CAD build for the part. Positions are in the model's coordinates, mm. Round coordinates to 2 decimals unless told otherwise and drop trailing zeros. Write each loop counter-clockwise with the first axis right and the second up, starting at its lowest first coordinate (ties: lowest second). Pieces come first, ordered by that corner, then holes. Notation, with made-up numbers: (46, 42) - (92, 42) arc R24 cw to (92, 57) - close; hole circle Ø11 at (52.25, -15). An arc over 180 degrees is marked (long way). Answer in a Markdown table with one row per item.
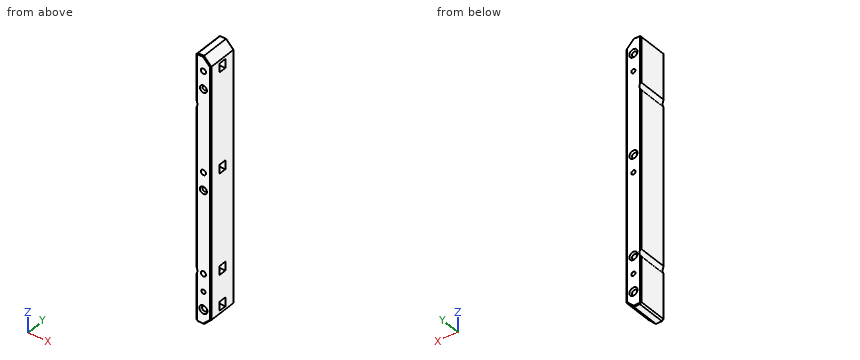
```python
from build123d import *

# Parameters (mm, degrees)
SKETCH1_W           = 10
SKETCH1_H           = 20
BOSS_EXTRUDE1_DEPTH = 90
SKETCH6_R           = 1.75
CUT_EXTRUDE4_DEPTH  = 93.330926563
SKETCH7_R           = 1.4
CUT_EXTRUDE5_DEPTH  = 93.330926563
CUT_EXTRUDE6_START  = -10
CUT_EXTRUDE6_DEPTH  = 2.5
CHAMFER2_SIZE       = 5
CHAMFER3_SIZE       = 1
CHAMFER4_SIZE       = 0.5
CHAMFER5_SIZE       = 0.5
SKETCH10_R          = 3.75
CUT_EXTRUDE7_DEPTH  = 93.330926563


with BuildPart() as part:
    # Sketch1 → Boss-Extrude1 (new, symmetric)
    with BuildSketch(Plane.XY):
        Rectangle(SKETCH1_W, SKETCH1_H)
    extrude(amount=BOSS_EXTRUDE1_DEPTH, both=True)

    # Sketch6 → Cut-Extrude4 (cut, through all)
    with BuildSketch(Plane.XZ.offset(10)):
        with Locations((0, 80)):
            Circle(SKETCH6_R)
        with Locations((0, -80)):
            Circle(SKETCH6_R)
        with Locations((0, 12)):
            Circle(SKETCH6_R)
        with Locations((0, -56)):
            Circle(SKETCH6_R)
    extrude(amount=-CUT_EXTRUDE4_DEPTH, mode=Mode.SUBTRACT)

    # Sketch7 → Cut-Extrude5 (cut, through all)
    with BuildSketch(Plane(origin=(0, 10, 0), x_dir=(1, 0, 0), z_dir=(0, 1, 0))):
        with Locations(Location((0, 68, 0), (0, 0, 270))):
            Circle(SKETCH7_R)
        with Locations(Location((0, 0, 0), (0, 0, 270))):
            Circle(SKETCH7_R)
        with Locations(Location((0, -68, 0), (0, 0, 270))):
            Circle(SKETCH7_R)
    extrude(amount=-CUT_EXTRUDE5_DEPTH, mode=Mode.SUBTRACT)

    # Sketch9 → Cut-Extrude6 (cut, symmetric)
    with BuildSketch(Plane(origin=(0, 10, 0), x_dir=(1, 0, 0), z_dir=(0, 1, 0)).offset(CUT_EXTRUDE6_START)):
        Polygon((1.732050808, -77), (-1.732050808, -77), (-3.464101615, -80), (-1.732050808, -83), (1.732050808, -83), (12.756943772, -83), (12.756943772, -77), align=None)
        Polygon((-3.464101615, 80), (-1.732050808, 77), (1.732050808, 77), (12.756943772, 77), (12.756943772, 83), (1.732050808, 83), (-1.732050808, 83), align=None)
        Polygon((1.732050808, -9), (-1.732050808, -9), (-3.464101615, -12), (-1.732050808, -15), (1.732050808, -15), (12.756943772, -15), (12.756943772, -9), align=None)
        Polygon((1.732050808, 59), (-1.732050808, 59), (-3.464101615, 56), (-1.732050808, 53), (1.732050808, 53), (12.756943772, 53), (12.756943772, 59), align=None)
    extrude(amount=CUT_EXTRUDE6_DEPTH, both=True, mode=Mode.SUBTRACT)

    # Chamfer2
    chamfer2_edges = [part.edges().sort_by_distance(p)[0] for p in [
        (5, 0, 90),
        (5, 0, -90),
    ]]
    chamfer(chamfer2_edges, length=CHAMFER2_SIZE)

    # Chamfer3
    chamfer3_edges = [part.edges().sort_by_distance(p)[0] for p in [
        (-1.75, 10, 80),
        (-1.75, 10, -56),
        (-1.75, 10, 12),
        (-1.75, 10, -80),
        (-1.75, -10, -80),
        (0, -10, -1.4),
        (0, -10, 66.6),
        (-5, 0, 90),
        (-5, 0, -90),
    ]]
    chamfer(chamfer3_edges, length=CHAMFER3_SIZE)

    # Chamfer4
    chamfer4_edges = [part.edges().sort_by_distance(p)[0] for p in [
        (5, -10, 0),
        (2.5, -10, 87.5),
        (2.5, -10, -87.5),
        (-2, -10, -90),
        (-2, -10, 90),
        (-5, -10, 0),
        (-4.5, -10, 89.5),
        (-4.5, -10, -89.5),
    ]]
    chamfer(chamfer4_edges, length=CHAMFER4_SIZE)

    # Chamfer5
    chamfer5_edges = [part.edges().sort_by_distance(p)[0] for p in [
        (5, 10, 0),
        (-2, 10, -90),
        (-2, 10, 90),
        (2.5, 10, 87.5),
        (2.5, 10, -87.5),
        (-5, 10, 0),
        (-4.5, 10, 89.5),
        (-4.5, 10, -89.5),
    ]]
    chamfer(chamfer5_edges, length=CHAMFER5_SIZE)

    # Sketch10 → Cut-Extrude7 (cut, through all)
    with BuildSketch(Plane.XZ.offset(10)):
        with Locations((-7.848531477, -55.883586947)):
            Circle(SKETCH10_R)
        with Locations((-7.848531477, 55.883586947)):
            Circle(SKETCH10_R)
    extrude(amount=-CUT_EXTRUDE7_DEPTH, mode=Mode.SUBTRACT)


solid = part.part
```
Q1. Flat gauge pins, fed straight in: pin 1 (4.5 mm diameter, centred on x = 0, z = 12, fed in from +Y); pin 2 (3 mm diameter, centred on x = 0, z = -80, fed in from +Y); pin 3 (4 mm diameter, centred on x = 3, y = 0.5, fed in from -Z); pin 4 (2.5 mm diameter, centred on x = 3, y = 1, fed in from -Z). Where does each tip first touch, or does it go through?
Computed:
| item | result |
|---|---|
| pin 1 | stops at y = 9.5 |
| pin 2 | passes through |
| pin 3 | stops at z = -89 |
| pin 4 | stops at z = -88.25 |
Q2. Drill centre lines: line 1 (X direction, y = 1, z = -68); line 2 (X direction, y = 4.5, z = 81.5); line 3 (Z direction, x = 3.5, y = 7.5). Where is each one in solid material? Low to high.
Computed:
| item | result |
|---|---|
| line 1 | x = -5 to -1.4, 1.4 to 5 |
| line 2 | x = -5 to -0.9, 0.9 to 5 |
| line 3 | z = -86.5 to 86.5 |
Q3. Saw through at A-A on y = 5.75. List the corners of the cut face in (x, z), then the cut area to 3 significant figures.
Computed:
| item | result |
|---|---|
| outline | (-5, -89) - (-4, -90) - (0, -90) - (5, -85) - (5, 85) - (0, 90) - (-4, 90) - (-5, 89) - (-5, 58.32) arc R3.75 cw to (-5, 53.44) - (-5, -53.44) arc R3.75 cw to (-5, -58.32) - close; hole circle Ø3.5 at (0, -80); hole circle Ø3.5 at (0, -56); hole circle Ø3.5 at (0, 12); hole circle Ø3.5 at (0, 80); hole circle Ø2.8 at (0, -68); hole circle Ø2.8 at (0, 0); hole circle Ø2.8 at (0, 68) |
| area | 1,710 mm2 |
